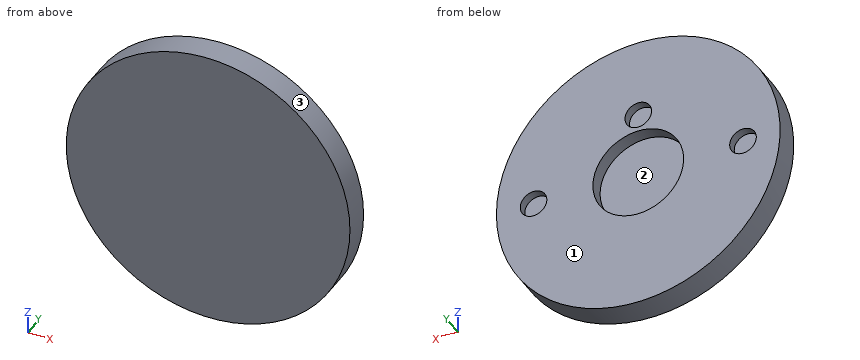
```python
from build123d import *

# Parameters (mm, degrees)
SKETCH1_R           = 101.6
BOSS_EXTRUDE1_DEPTH = 19.05
SKETCH2_R           = 32.5
CUT_EXTRUDE1_DEPTH  = 10
SKETCH4_R           = 9.525
CUT_EXTRUDE3_DEPTH  = 6.35
SKETCH5_R           = 9.525
CUT_EXTRUDE4_DEPTH  = 6.35
SKETCH6_R           = 9.525
CUT_EXTRUDE5_DEPTH  = 6.35


with BuildPart() as part:
    # Sketch1 → Boss-Extrude1 (new body)
    with BuildSketch(Plane(origin=(0, 0, 0), x_dir=(1, 0, 0), z_dir=(0, 1, 0))):
        Circle(SKETCH1_R)
    extrude(amount=BOSS_EXTRUDE1_DEPTH)

    # Sketch2 → Cut-Extrude1 (cut)
    with BuildSketch(Plane(origin=(0, 19.05, 0), x_dir=(1, 0, 0), z_dir=(0, 1, 0))):
        Circle(SKETCH2_R)
    extrude(amount=-CUT_EXTRUDE1_DEPTH, mode=Mode.SUBTRACT)

    # Sketch4 → Cut-Extrude3 (cut)
    with BuildSketch(Plane(origin=(0, 19.05, 0), x_dir=(1, 0, 0), z_dir=(0, 1, 0))):
        with Locations((-75, 0)):
            Circle(SKETCH4_R)
    extrude(amount=-CUT_EXTRUDE3_DEPTH, mode=Mode.SUBTRACT)

    # Sketch5 → Cut-Extrude4 (cut)
    with BuildSketch(Plane(origin=(0, 19.05, 0), x_dir=(1, 0, 0), z_dir=(0, 1, 0))):
        with Locations((75, 0)):
            Circle(SKETCH5_R)
    extrude(amount=-CUT_EXTRUDE4_DEPTH, mode=Mode.SUBTRACT)

    # Sketch6 → Cut-Extrude5 (cut)
    with BuildSketch(Plane(origin=(0, 19.05, 0), x_dir=(1, 0, 0), z_dir=(0, 1, 0))):
        with Locations((0, -45)):
            Circle(SKETCH6_R)
    extrude(amount=-CUT_EXTRUDE5_DEPTH, mode=Mode.SUBTRACT)


solid = part.part
```
Read the model definition and answer for the solid it produces. Units are mm, in the model's axes. Face numbers are marked on the shaded views. Give positions to 0.01 mm unless a question says otherwise; leave off trailing zeros. Write each loop counter-clockwise with the first axis right and the second up, starting at its lowest first coordinate (ties: lowest second). Pieces come first, ordered by that corner, then holes. Notation, with made-up numbers: (53.5, -2.75) -> (78.5, -2.75) arc R20 ccw to (78.5, 9.25) -> close; hole circle Ø6 at (79, 6.5). An arc over 180 degrees is marked (long way). Answer in a Markdown table with one row per item.
1) Determine the mould class of the marked faces 1, 2 and 3 for opening direction X: released by +X, released by -X, zero draft, split by the parting line, or undercut.
Results list:
| item | result |
|---|---|
| face 1 | zero draft |
| face 2 | undercut |
| face 3 | split by the parting line |
2) Section D-D on y = 2.75 is taken. Give the vertices of the cut face in (x, z).
Results list:
| item | result |
|---|---|
| outline | circle Ø203.2 at (0, 0) |
3) Straight lines are drawn through the part: line 1 (X direction, y = 14.5, z = 0) (3 decimals); line 2 (Z direction, x = 0, y = 15.75) (3 decimals); line 3 (Y direction, x = -3.5, z = -21). For each, find the intervals that lie inside material, in ascending order. Write a range as [from, to].
Results list:
| item | result |
|---|---|
| line 1 | [-101.6, -84.525], [-65.475, -32.5], [32.5, 65.475], [84.525, 101.6] |
| line 2 | [-101.6, -32.5], [32.5, 35.475], [54.525, 101.6] |
| line 3 | [0, 9.05] |
4) Each of these flat-tipped pins is pushed along its axis until it touches: pin 1 Ø1 at (y, z) = (4, 38) entering from -X; pin 2 Ø5 at (x, y) = (7, 10.5) entering from +Z; pin 3 Ø3 at (x, y) = (-64.5, 8.5) entering from +Z. Where does it stop, or does it pass through?
Results list:
| item | result |
|---|---|
| pin 1 | x = -94.43 |
| pin 2 | z = 101.5 |
| pin 3 | z = 79.71 |
5) Section C-C on z = 0 is taken. Give the vertices of the cut face in (x, y) (3 decimals), plus the area to 3 significant figures.
Results list:
| item | result |
|---|---|
| outline | (-101.6, 0) -> (101.6, 0) -> (101.6, 19.05) -> (84.525, 19.05) -> (84.525, 12.7) -> (65.475, 12.7) -> (65.475, 19.05) -> (32.5, 19.05) -> (32.5, 9.05) -> (-32.5, 9.05) -> (-32.5, 19.05) -> (-65.475, 19.05) -> (-65.475, 12.7) -> (-84.525, 12.7) -> (-84.525, 19.05) -> (-101.6, 19.05) -> close |
| area | 2,980 mm^2 |
6) Section A-A on y = 16 is taken. Give the vertices of the cut face in (x, z) (3 decimals).
Results list:
| item | result |
|---|---|
| outline | circle Ø203.2 at (0, 0); hole circle Ø19.05 at (-75, 0); hole circle Ø65 at (0, 0); hole circle Ø19.05 at (0, 45); hole circle Ø19.05 at (75, 0) |
7) Section B-B on x = 0 is taken. Give the vertices of the cut face in (y, z) (3 decimals), plus the area to 3 significant figures.
Results list:
| item | result |
|---|---|
| outline | (0, -101.6) -> (19.05, -101.6) -> (19.05, -32.5) -> (9.05, -32.5) -> (9.05, 32.5) -> (19.05, 32.5) -> (19.05, 35.475) -> (12.7, 35.475) -> (12.7, 54.525) -> (19.05, 54.525) -> (19.05, 101.6) -> (0, 101.6) -> close |
| area | 3,100 mm^2 |
